Check sheet for the modelled part. Datum: model origin and axes. Units: mm. A direction names the side the tool comes from. Round coordinates to 2 decimals unless told otherwise and drop trailing zeros. Write each loop counter-clockwise with the first axis right and the second up, starting at its lowest first coordinate (ties: lowest second). Pieces come first, ordered by that corner, then holes.
Item 1: Section check B-B, the plane z = 8. Record the cut outline in (x, y).
Item 2: Section check C-C, the plane y = 2.5. Record the cut outline in (x, z), plus the area to 3 significant figures.
Item 3: Section check D-D, the plane x = -4. Record the cut outline in (y, z), plus the area to 3 significant figures.
Item 4: Depth check by flat-ended pin: pin 1 (6 mm diameter, centred on y = 1.5, z = 21.5, fed in from +X); pin 2 (1.5 mm diameter, centred on x = -0.5, z = 24.5, fed in from +Y); pin 3 (4 mm diameter, centred on x = -4.5, z = 16, fed in from +Y). Enter the tip coordinate at first touch or a pass-through.
Item 5: Section check A-A, the plane y = 0. Record the cut outline in (x, z).
Item 6: Material ranges on line 1 along Z through (x, y) = (0, -1.75); line 2 along Z through (x, y) = (-4, 2.25); line 3 along X through (y, z) = (0, 7), recorded low to high.
Item 7: Set-up check for faces 4 (the flat face through (-2.881, 5.334, 47.479)), 5 (the flat face through (3, -3, 46)): record each of +Z, -Z, +X, -X, +Y, -Y from which the full face is reachable in a straight line by a thin tool's end or side.
Item 8: Release check for a two-part mould opening along X. For faces 1 (the flat face through (0, 0, -3)), 2 (the flat face through (2.881, -5.334, 47.479)), 3 (the cylindrical face through (-0.19, -0.05, -0.65)) record: pulls with the +X half, pulls with the -X half, needs draft (parallel to the pull), parting line crosses it, or undercut.
from build123d import *

# Parameters (mm, degrees)
SKETCH1_R               = 3.5
BOSS_EXTRUDE1_DEPTH     = 46
BOSS_EXTRUDE2_DEPTH     = 3
BOSS_EXTRUDE3_START     = 3
SKETCH3_R               = 3.5
BOSS_EXTRUDE3_DEPTH     = 3
CUT_EXTRUDE2_DEPTH      = 13
CUT_EXTRUDE2_DEPTH_BACK = 15
SKETCH4_R               = 0.5


with BuildPart() as part:
    # Sketch1 → Boss-Extrude1 (new body)
    with BuildSketch(Plane.XY):
        Circle(SKETCH1_R)
    extrude(amount=BOSS_EXTRUDE1_DEPTH)

    # Sketch2 → Boss-Extrude2 (add)
    with BuildSketch(Plane.XY.offset(46)):
        Polygon((0.14203789, 6.998558797), (-5.989910763, 3.62228782), (-6.131948653, -3.376270977), (-0.14203789, -6.998558797), (5.989910763, -3.62228782), (6.131948653, 3.376270977), align=None)
    extrude(amount=BOSS_EXTRUDE2_DEPTH)

    # Sketch3 → Boss-Extrude3 (add)
    with BuildSketch(Plane(origin=(0, 0, 0), x_dir=(-1, 0, 0), z_dir=(0, 0, -1)).offset(BOSS_EXTRUDE3_START)):
        Circle(SKETCH3_R)
    extrude(amount=-BOSS_EXTRUDE3_DEPTH)

    # Sketch4 → Cut-Extrude2 (cut, two sides: drawn at the far end of the back side and taken through both)
    with BuildSketch(Plane(origin=(0, 0, 0), x_dir=(1, 0, 0), z_dir=(0, 1, 0)).offset(-CUT_EXTRUDE2_DEPTH_BACK)):
        with Locations(Location((0, 1.112079682, 0), (0, 0, 270))):
            Circle(SKETCH4_R)
    extrude(amount=CUT_EXTRUDE2_DEPTH + CUT_EXTRUDE2_DEPTH_BACK, mode=Mode.SUBTRACT)


solid = part.part
Values found:
1. outline: circle Ø7 at (0, 0)
2. outline: (-6.01, 46) - (-2.45, 46) - (-2.45, -3) - (2.45, -3) - (2.45, 46) - (6.11, 46) - (6.11, 49) - (-6.01, 49) - close; hole circle Ø1 at (0, -1.11)
2. area: 276 mm2
3. outline: (-4.67, 46) - (4.72, 46) - (4.72, 49) - (-4.67, 49) - close
3. area: 28.2 mm2
4. pin 1: stops at x = 3.5
4. pin 2: stops at y = 3.5
4. pin 3: stops at y = 2.45
5. outline: (-6.06, 46) - (-3.5, 46) - (-3.5, -3) - (3.5, -3) - (3.5, 46) - (6.06, 46) - (6.06, 49) - (-6.06, 49) - close; hole circle Ø1 at (0, -1.11)
6. line 1: z = -3 to -1.61, -0.61 to 49
6. line 2: z = 46 to 49
6. line 3: x = -3.5 to 3.5
7. face 4: +Z, -Z, -X, +Y
7. face 5: -Z
8. face 1: needs draft
8. face 2: pulls with the +X half
8. face 3: undercut
